```python
from build123d import *

# Parameters (mm, degrees)
SKETCH021_R     = 2.55
SKETCH021_W     = 33
SKETCH021_H     = 33
SKETCH021_W_2   = 62
SKETCH021_H_2   = 14.5
PAD013_DEPTH    = 17
FILLET010_R     = 30
FILLET011_R     = 3
SKETCH023_W     = 178
SKETCH023_H     = 19.5
POCKET006_DEPTH = 7.4
SKETCH024_R     = 0.9
POCKET007_DEPTH = 6
SKETCH025_W     = 72
SKETCH025_H     = 34
POCKET008_DEPTH = 3
POCKET012_DEPTH = 10
SKETCH028_R     = 1.25
POCKET013_DEPTH = 7
SKETCH030_R     = 0.9
POCKET014_DEPTH = 8


with BuildPart() as part:
    # Sketch021 → Pad013 (new body)
    with BuildSketch(Plane.XY):
        with BuildLine():
            Line((-90, -38.5), (-90, 17.5))
            ThreePointArc((90, 17.5), (0, 30.595035), (-90, 17.5))
            Line((90, 17.5), (90, -38.5))
            Line((90, -38.5), (-90, -38.5))
        make_face()
        with Locations((-45, 2.5)):
            Circle(SKETCH021_R, mode=Mode.SUBTRACT)
        with Locations((-45, -5)):
            Circle(SKETCH021_R, mode=Mode.SUBTRACT)
        with Locations((-45, -12.5)):
            Circle(SKETCH021_R, mode=Mode.SUBTRACT)
        with Locations((-45, 20.135045)):
            Circle(SKETCH021_R, mode=Mode.SUBTRACT)
        with Locations((-35, 21.92157)):
            Circle(SKETCH021_R, mode=Mode.SUBTRACT)
        with Locations((-25, 23.252201)):
            Circle(SKETCH021_R, mode=Mode.SUBTRACT)
        with Locations((-15, 24.134956)):
            Circle(SKETCH021_R, mode=Mode.SUBTRACT)
        with Locations((-5, 24.575048)):
            Circle(SKETCH021_R, mode=Mode.SUBTRACT)
        with Locations((5, 24.575048)):
            Circle(SKETCH021_R, mode=Mode.SUBTRACT)
        with Locations((15, 24.134956)):
            Circle(SKETCH021_R, mode=Mode.SUBTRACT)
        with Locations((25, 23.252201)):
            Circle(SKETCH021_R, mode=Mode.SUBTRACT)
        with Locations((35, 21.92157)):
            Circle(SKETCH021_R, mode=Mode.SUBTRACT)
        with Locations((45, 20.135045)):
            Circle(SKETCH021_R, mode=Mode.SUBTRACT)
        with Locations((45, 2.5)):
            Circle(SKETCH021_R, mode=Mode.SUBTRACT)
        with Locations((45, -12.5)):
            Circle(SKETCH021_R, mode=Mode.SUBTRACT)
        with Locations((45, -5)):
            Circle(SKETCH021_R, mode=Mode.SUBTRACT)
        Rectangle(SKETCH021_W, SKETCH021_H, mode=Mode.SUBTRACT)
        with Locations((-45, -27.75)):
            Rectangle(SKETCH021_W_2, SKETCH021_H_2, mode=Mode.SUBTRACT)
        with Locations((45, -27.75)):
            Rectangle(SKETCH021_W_2, SKETCH021_H_2, mode=Mode.SUBTRACT)
    extrude(amount=PAD013_DEPTH)

    # Fillet010
    fillet010_edges = [part.edges().sort_by_distance(p)[0] for p in [
        (90, 17.5, 8.5),
        (-90, 17.5, 8.5),
    ]]
    fillet(fillet010_edges, radius=FILLET010_R)

    # Fillet011
    fillet011_edges = [part.edges().sort_by_distance(p)[0] for p in [
        (-90, -38.5, 8.5),
        (90, -38.5, 8.5),
    ]]
    fillet(fillet011_edges, radius=FILLET011_R)

    # Sketch023 (on Face33 of Pad013) → Pocket006 (cut)
    with BuildSketch(Plane(origin=(0, 0, 0), x_dir=(1, 0, 0), z_dir=(0, 0, -1))):
        with Locations((0, 26.75)):
            Rectangle(SKETCH023_W, SKETCH023_H)
    extrude(amount=-POCKET006_DEPTH, mode=Mode.SUBTRACT)

    # Sketch024 (on Face43 of Pocket006) → Pocket007 (cut)
    with BuildSketch(Plane(origin=(0, 0, 7.4), x_dir=(1, 0, 0), z_dir=(0, 0, -1))):
        with Locations((-82.5, 32.95)):
            Circle(SKETCH024_R)
        with Locations((-6, 23.95)):
            Circle(SKETCH024_R)
        with Locations((9.7, 23.95)):
            Circle(SKETCH024_R)
        with Locations((86.2, 32.95)):
            Circle(SKETCH024_R)
    extrude(amount=-POCKET007_DEPTH, mode=Mode.SUBTRACT)

    # Sketch025 (on Face2 of Pocket007) → Pocket008 (cut)
    with BuildSketch(Plane(origin=(0, 0, 0), x_dir=(1, 0, 0), z_dir=(0, 0, -1))):
        Rectangle(SKETCH025_W, SKETCH025_H)
    extrude(amount=-POCKET008_DEPTH, mode=Mode.SUBTRACT)

    # Sketch029 (on Face46 of Pocket008) → Pocket012 (cut)
    with BuildSketch(Plane(origin=(0, 0, 3), x_dir=(1, 0, 0), z_dir=(0, 0, -1))):
        Polygon((-27, 17), (-27, 10), (-34, 10), (-34, -10), (-27, -10), (-27, -17), (27, -17), (27, -10), (34, -10), (34, 10), (27, 10), (27, 17), align=None)
    extrude(amount=-POCKET012_DEPTH, mode=Mode.SUBTRACT)

    # Sketch028 (on Face2 of Pocket012) → Pocket013 (cut)
    with BuildSketch(Plane(origin=(0, 0, 0), x_dir=(1, 0, 0), z_dir=(0, 0, -1))):
        with Locations((-72, -14)):
            Circle(SKETCH028_R)
        with Locations((72, -14)):
            Circle(SKETCH028_R)
        Polygon((-84.275394, 19.474852), (-84.275394, 4.973012), (-52.122028, -24.818211), (-29.766602, -27.995476), (-10.059475, -29.217621), (0, -29.217621), (11.128853, -29.217621), (29.766602, -27.995476), (52.122028, -24.818211), (84.122627, 4.973012), (84.122627, 19.355327), (35.69899, 19.355327), (35.69899, -14.760202), (31.141516, -16.974091), (0, -16.974091), (-31.141516, -16.974091), (-35.69899, -14.760202), (-35.69899, 19.474852), align=None)
    extrude(amount=-POCKET013_DEPTH, mode=Mode.SUBTRACT)

    # Sketch030 (on Face61 of Pocket013) → Pocket014 (cut)
    with BuildSketch(Plane(origin=(0, 0, 3), x_dir=(1, 0, 0), z_dir=(0, 0, -1))):
        with Locations((-32, 13.4)):
            Circle(SKETCH030_R)
        with Locations((-32, -13.4)):
            Circle(SKETCH030_R)
        with Locations((32, -13.4)):
            Circle(SKETCH030_R)
        with Locations((32, 13.4)):
            Circle(SKETCH030_R)
    extrude(amount=-POCKET014_DEPTH, mode=Mode.SUBTRACT)


solid = part.part
```
Check sheet for the modelled part. Datum: model origin and axes. Units: mm. A direction names the side the tool comes from. Round coordinates to 2 decimals unless told otherwise and drop trailing zeros. Order: outer loops, then holes, each group sorted by start corner. A loop starts at its lowest first (then second) coordinate and runs counter-clockwise, first axis right, second up. Notation, with made-up numbers: M 23.25,9.5 L 56.25,9.5 A21 ccw 56.25,24.5 Z; hole C 28,26.25 d8. An arc over 180 degrees is marked long. Answer in a Markdown table with one row per item.
(1) Draft check along X on faces 3 (the flat face through (14, -28, 12)), 4 (the cylindrical face through (-83.51, 12.86, 8.62)). Enter one of: +X half, -X half, draft (parallel to the pull), parting line (faces both ways), or undercut.
Findings:
| item | result |
|---|---|
| face 3 | undercut |
| face 4 | -X half |
(2) Section check C-C on x = 25. Record the boundary of the cut face in (y, z), plus the area to 3 significant figures.
Findings:
| item | result |
|---|---|
| outline | M -38.5,0 L -36.5,0 L -36.5,7.4 L -35,7.4 L -35,17 L -38.5,17 Z; M -20.5,7.4 L -17,7.4 L -17,13 L 17,13 L 17,7 L 20.7,7 L 20.7,17 L -20.5,17 Z; M 25.8,7 L 28.31,7 L 28.31,0 L 29.6,0 L 29.6,17 L 25.8,17 Z |
| area | 302 mm^2 |
(3) Gauge pin test, flat ends, axial feed: pin 1 (1.2 mm diameter, centred on y = -3, z = 15.5, fed in from +X); pin 2 (8 mm diameter, centred on x = 32, y = 3, fed in from -Z); pin 3 (2 mm diameter, centred on x = 37.5, y = 12, fed in from -Z); pin 4 (4 mm diameter, centred on x = -45, y = 2.5, fed in from -Z). Record the tip position at first contact, or that the pin passes through.
Findings:
| item | result |
|---|---|
| pin 1 | stops at x = 89.92 |
| pin 2 | stops at z = 3 |
| pin 3 | stops at z = 7 |
| pin 4 | passes through |
(4) Section check B-B on y = 8. Record the boundary of the cut face in (x, z), plus the area to 3 significant figures.
Findings:
| item | result |
|---|---|
| outline | M -86.65,0 L -70.27,0 L -70.27,7 L -35.7,7 L -35.7,3 L -34,3 L -34,13 L -16.5,13 L -16.5,17 L -86.65,17 Z; M 16.5,13 L 34,13 L 34,3 L 35.7,3 L 35.7,7 L 70.19,7 L 70.19,0 L 86.65,0 L 86.65,17 L 16.5,17 Z |
| area | 1,440 mm^2 |
(5) Set-up check for faces 1 (the flat face through (0, 17, 10)), 2 (the flat face through (0, -16.5, 15)): record each of +Z, -Z, +X, -X, +Y, -Y from which the full face is reachable in a straight line by a thin tool's end or side.
Findings:
| item | result |
|---|---|
| face 1 | -Z |
| face 2 | +Z, -Z |
(6) Section check A-A on x = -63.5. Record the boundary of the cut face in (y, z).
Findings:
| item | result |
|---|---|
| outline | M -38.5,0 L -36.5,0 L -36.5,7.4 L -35,7.4 L -35,17 L -38.5,17 Z; M -20.5,7.4 L -17,7.4 L -17,7 L 14.28,7 L 14.28,0 L 24.15,0 L 24.15,17 L -20.5,17 Z |
(7) Section check D-D on x = 63. Record the boundary of the cut face in (y, z).
Findings:
| item | result |
|---|---|
| outline | M -38.5,0 L -36.5,0 L -36.5,7.4 L -35,7.4 L -35,17 L -38.5,17 Z; M -20.5,7.4 L -17,7.4 L -17,7 L 14.69,7 L 14.69,0 L 24.25,0 L 24.25,17 L -20.5,17 Z |
(8) Material ranges on line 1 along X through (y, z) = (-23.95, 11.05); line 2 along X through (y, z) = (-13.4, 6.5); line 3 along X through (y, z) = (-13.4, 7.5), recorded low to high. Write a range as from..to.
Findings:
| item | result |
|---|---|
| line 1 | x = -90..-76, -14..-6.9, -5.1..8.8, 10.6..14, 76..90 |
| line 2 | x = -90..-84.28, -35.7..-32.9, -31.1..-27, 27..31.1, 32.9..35.7, 84.12..90 |
| line 3 | x = -90..-47.39, -42.61..-32.9, -31.1..-27, 27..31.1, 32.9..42.61, 47.39..90 |
